Source: CAD feature listing. Evaluate the final solid. Frame: model axes, mm. A direction names the side the tool comes from. Give positions to 0.01 mm unless a question says otherwise; leave off trailing zeros. Order: outer loops, then holes, each group sorted by start corner. A loop starts at its lowest first (then second) coordinate and runs counter-clockwise, first axis right, second up. Notation, with made-up numbers: M 28,-14 L 45,-14 A12 cw 45,2 Z; hole C 9.25,20 d2. An arc over 180 degrees is marked long. Answer as a JSON object with one key per item and string values. Group by question number.
1. Section query C-C (z = -40.5). Output: boundary loops of the cut face in (x, y), plus the area to 3 significant figures.
2. Section query B-B (x = 20). Output: boundary loops of the cut face in (y, z).
3. Section query D-D (y = -7.5). Output: boundary loops of the cut face in (x, z).
4. Material intervals for L1, parallel to X at y = 2.3, z = 35.5; L2, parallel to Z at x = 40, y = 1.95; L3, parallel to X at y = 1.65, z = 90, sorted ascending. Write a range as [from, to].
5. Section query A-A (x = 0). Output: boundary loops of the cut face in (y, z).
6. Set-up query: faces 1 (the flat face through (0, -5, -95.5)), 2 (the cylindrical face through (20, 2, 65)), 3 (the flat face through (-10, -5, -93)), 4 (the flat face through (10, -5, -93)). Return all of +Z, -Z, +X, -X, +Y, -Y with unobstructed straight access to the full face (end or side cutting, diameter ignored); none if empty.
7. Pin query (flat end, axial travel): P1, Ø3.5, axis at x = 88, y = 1, coming from the -Z side; P2, Ø4, axis at x = 59, z = 69, coming from the -Y side; P3, Ø3.5, axis at x = -89, y = 2, coming from the -Z side. Return the tip coordinate at first contact, or that it passes through.
8. Pull-direction query (Z, two-part tool) for faces 5 (the flat face through (0, -5, -90.499)), 6 (the cylindrical face through (-20, 2, 15)), 7 (the flat face through (-1, 3, -24)); classes: +Z half, -Z half, draft (parallel to the pull), parting line (faces both ways), or undercut.
from build123d import *

# Parameters (mm, degrees)
SKETCH1_W               = 200
SKETCH1_H               = 200
BOSS_EXTRUDE1_DEPTH     = 3
CUT_EXTRUDE1_START      = -4
SKETCH2_W               = 30
SKETCH2_H               = 70
CUT_EXTRUDE1_DEPTH      = 14
SKETCH4_W               = 3
SKETCH4_H               = 5
CUT_EXTRUDE2_DEPTH      = 4
SKETCH5_W               = 3
SKETCH5_H               = 5
CUT_EXTRUDE3_DEPTH      = 4
CUT_EXTRUDE4_DEPTH      = 4
FILLET1_R               = 45
SKETCH9_R               = 1.5
SKETCH9_W               = 22
SKETCH9_H               = 3
CUT_EXTRUDE7_DEPTH      = 4
SKETCH11_R              = 1.5
CUT_EXTRUDE8_DEPTH      = 4
SKETCH10_R              = 1.5
CUT_EXTRUDE9_DEPTH      = 4
LPATTERN1_COUNT         = 2
LPATTERN1_PITCH         = 40
LPATTERN1_COUNT_DIR2    = 2
LPATTERN1_PITCH_DIR2    = 20
SKETCH13_R              = 1.5
CUT_EXTRUDE10_DEPTH     = 4
MIRROR1_COPY_1_SKETCH_R = 1.5
MIRROR1_COPY_1_DEPTH    = 4
MIRROR1_COPY_2_SKETCH_R = 1.5
MIRROR1_COPY_2_DEPTH    = 4
MIRROR1_COPY_3_SKETCH_R = 1.5
MIRROR1_COPY_3_DEPTH    = 4
FILLET2_R               = 0.5
SKETCH23_W              = 20
SKETCH23_H              = 5.000586006
BOSS_EXTRUDE7_DEPTH     = 10
SKETCH26_R              = 1.5
CUT_EXTRUDE11_DEPTH     = 10
SKETCH27_R              = 2.5
CUT_EXTRUDE12_DEPTH     = 10
SKETCH28_R              = 1
CUT_EXTRUDE13_DEPTH     = 10


with BuildPart() as part:
    # Sketch1 → Boss-Extrude1 (new body)
    with BuildSketch(Plane(origin=(0, 0, 0), x_dir=(1, 0, 0), z_dir=(0, 1, 0))):
        Rectangle(SKETCH1_W, SKETCH1_H)
    extrude(amount=BOSS_EXTRUDE1_DEPTH)

    # Sketch2 → Cut-Extrude1 (cut)
    with BuildSketch(Plane(origin=(0, 3, 0), x_dir=(1, 0, 0), z_dir=(0, 1, 0)).offset(CUT_EXTRUDE1_START)):
        with Locations((-85, -25)):
            Rectangle(SKETCH2_W, SKETCH2_H)
    cut_extrude1 = extrude(amount=CUT_EXTRUDE1_DEPTH, mode=Mode.SUBTRACT)

    # Sketch4 → Cut-Extrude2 (cut, through all)
    with BuildSketch(Plane(origin=(0, 3, 0), x_dir=(1, 0, 0), z_dir=(0, 1, 0))):
        with Locations((-88.5, -89.5)):
            Rectangle(SKETCH4_W, SKETCH4_H)
    cut_extrude2 = extrude(amount=-CUT_EXTRUDE2_DEPTH, mode=Mode.SUBTRACT)

    # Sketch5 → Cut-Extrude3 (cut, through all)
    with BuildSketch(Plane(origin=(0, 3, 0), x_dir=(1, 0, 0), z_dir=(0, 1, 0))):
        with Locations((-88.5, 57.5)):
            Rectangle(SKETCH5_W, SKETCH5_H)
    cut_extrude3 = extrude(amount=-CUT_EXTRUDE3_DEPTH, mode=Mode.SUBTRACT)

    # Sketch7 → Cut-Extrude4 (cut, through all)
    with BuildSketch(Plane(origin=(0, 3, 0), x_dir=(1, 0, 0), z_dir=(0, 1, 0))):
        with BuildLine():
            Line((-30, -55), (-30, -25))
            ThreePointArc((-30, -25), (-20, -15), (-10, -25))
            Line((-10, -25), (-10, -55))
            ThreePointArc((-10, -55), (-20, -65), (-30, -55))
        make_face()
    cut_extrude4 = extrude(amount=-CUT_EXTRUDE4_DEPTH, mode=Mode.SUBTRACT)

    # Fillet1
    fillet1_edges = [part.edges().sort_by_distance(p)[0] for p in [
        (-100, 1.5, -100),
        (100, 1.5, -100),
    ]]
    fillet(fillet1_edges, radius=FILLET1_R)

    # Sketch9 → Cut-Extrude7 (cut, through all)
    with BuildSketch(Plane(origin=(0, 3, 0), x_dir=(1, 0, 0), z_dir=(0, 1, 0))):
        with Locations((-60, -90)):
            Circle(SKETCH9_R)
        with BuildLine():
            Line((-30, 80), (30, 80))
            ThreePointArc((30, 80), (35, 75), (30, 70))
            Line((30, 70), (-30, 70))
            ThreePointArc((-30, 70), (-35, 75), (-30, 80))
        make_face()
        with Locations((0, 88.5)):
            Rectangle(SKETCH9_W, SKETCH9_H)
    cut_extrude7 = extrude(amount=-CUT_EXTRUDE7_DEPTH, mode=Mode.SUBTRACT)

    # Sketch11 → Cut-Extrude8 (cut, through all)
    with BuildSketch(Plane(origin=(0, 3, 0), x_dir=(1, 0, 0), z_dir=(0, 1, 0))):
        with Locations((-45, 50)):
            Circle(SKETCH11_R)
    cut_extrude8 = extrude(amount=-CUT_EXTRUDE8_DEPTH, mode=Mode.SUBTRACT)

    # Sketch10 → Cut-Extrude9 (cut, through all)
    with BuildSketch(Plane(origin=(0, 3, 0), x_dir=(1, 0, 0), z_dir=(0, 1, 0))):
        with Locations((-60, -60)):
            Circle(SKETCH10_R)
    cut_extrude9 = extrude(amount=-CUT_EXTRUDE9_DEPTH, mode=Mode.SUBTRACT)

    # LPattern1: Cut-Extrude9 2 × 2
    with Locations(*[(j * LPATTERN1_PITCH_DIR2, 0, -i * LPATTERN1_PITCH) for i in range(LPATTERN1_COUNT) for j in range(LPATTERN1_COUNT_DIR2) if (i, j) != (0, 0)]):
        add(cut_extrude9, mode=Mode.SUBTRACT)

    # Sketch13 → Cut-Extrude10 (cut, through all)
    with BuildSketch(Plane(origin=(0, 3, 0), x_dir=(1, 0, 0), z_dir=(0, 1, 0))):
        with Locations((-60, 28)):
            Circle(SKETCH13_R)
    cut_extrude10 = extrude(amount=-CUT_EXTRUDE10_DEPTH, mode=Mode.SUBTRACT)

    # Mirror1: Cut-Extrude7, Cut-Extrude10, Cut-Extrude9, Cut-Extrude8, Cut-Extrude4, Cut-Extrude3, Cut-Extrude2, Cut-Extrude1 across plane
    add(cut_extrude7.mirror(Plane(origin=(0, 0, 0), x_dir=(0, 0, 1), z_dir=(1, 0, 0))), mode=Mode.SUBTRACT)
    add(cut_extrude10.mirror(Plane(origin=(0, 0, 0), x_dir=(0, 0, 1), z_dir=(1, 0, 0))), mode=Mode.SUBTRACT)
    add(cut_extrude9.mirror(Plane(origin=(0, 0, 0), x_dir=(0, 0, 1), z_dir=(1, 0, 0))), mode=Mode.SUBTRACT)
    add(cut_extrude8.mirror(Plane(origin=(0, 0, 0), x_dir=(0, 0, 1), z_dir=(1, 0, 0))), mode=Mode.SUBTRACT)
    add(cut_extrude4.mirror(Plane(origin=(0, 0, 0), x_dir=(0, 0, 1), z_dir=(1, 0, 0))), mode=Mode.SUBTRACT)
    add(cut_extrude3.mirror(Plane(origin=(0, 0, 0), x_dir=(0, 0, 1), z_dir=(1, 0, 0))), mode=Mode.SUBTRACT)
    add(cut_extrude2.mirror(Plane(origin=(0, 0, 0), x_dir=(0, 0, 1), z_dir=(1, 0, 0))), mode=Mode.SUBTRACT)
    add(cut_extrude1.mirror(Plane(origin=(0, 0, 0), x_dir=(0, 0, 1), z_dir=(1, 0, 0))), mode=Mode.SUBTRACT)

    # Mirror1 copy 1 sketch → Mirror1 copy 1 (cut, through all)
    with BuildSketch(Plane(origin=(-20, 3, 0), x_dir=(-1, 0, 0), z_dir=(0, 1, 0))):
        with Locations((-60, 60)):
            Circle(MIRROR1_COPY_1_SKETCH_R)
    extrude(amount=-MIRROR1_COPY_1_DEPTH, mode=Mode.SUBTRACT)

    # Mirror1 copy 2 sketch → Mirror1 copy 2 (cut, through all)
    with BuildSketch(Plane(origin=(0, 3, -40), x_dir=(-1, 0, 0), z_dir=(0, 1, 0))):
        with Locations((-60, 60)):
            Circle(MIRROR1_COPY_2_SKETCH_R)
    extrude(amount=-MIRROR1_COPY_2_DEPTH, mode=Mode.SUBTRACT)

    # Mirror1 copy 3 sketch → Mirror1 copy 3 (cut, through all)
    with BuildSketch(Plane(origin=(-20, 3, -40), x_dir=(-1, 0, 0), z_dir=(0, 1, 0))):
        with Locations((-60, 60)):
            Circle(MIRROR1_COPY_3_SKETCH_R)
    extrude(amount=-MIRROR1_COPY_3_DEPTH, mode=Mode.SUBTRACT)

    # Fillet2
    fillet2_edges = [part.edges().sort_by_distance(p)[0] for p in [
        (100, 3, 80),
        (100, 3, -32.5),
        (-100, 3, 80),
        (70, 3, 25),
        (85, 3, 60),
        (85, 3, -10),
        (-70, 3, 25),
        (-85, 3, -10),
        (-85, 3, 60),
        (0, 3, 100),
        (0, 3, -100),
        (-100, 3, -32.5),
        (-86.819805153, 3, -86.819805153),
        (86.819805153, 3, -86.819805153),
    ]]
    fillet(fillet2_edges, radius=FILLET2_R)

    # Sketch23 → Boss-Extrude7 (add)
    with BuildSketch(Plane.XZ):
        with Locations((0, -92.999706997)):
            Rectangle(SKETCH23_W, SKETCH23_H)
    extrude(amount=BOSS_EXTRUDE7_DEPTH)

    # Sketch26 → Cut-Extrude11 (cut)
    with BuildSketch(Plane(origin=(0, 3, 0), x_dir=(1, 0, 0), z_dir=(0, 1, 0))):
        with Locations((24, 45.74141283)):
            Circle(SKETCH26_R)
        with Locations((-24, 45.74141283)):
            Circle(SKETCH26_R)
    extrude(amount=-CUT_EXTRUDE11_DEPTH, mode=Mode.SUBTRACT)

    # Sketch27 → Cut-Extrude12 (cut)
    with BuildSketch(Plane(origin=(0, 3, 0), x_dir=(1, 0, 0), z_dir=(0, 1, 0))):
        Circle(SKETCH27_R)
    extrude(amount=-CUT_EXTRUDE12_DEPTH, mode=Mode.SUBTRACT)

    # Sketch28 → Cut-Extrude13 (cut)
    with BuildSketch(Plane(origin=(0, 3, 0), x_dir=(1, 0, 0), z_dir=(0, 1, 0))):
        with Locations((-62.25, -35.5)):
            Circle(SKETCH28_R)
        with Locations((62.25, -35.5)):
            Circle(SKETCH28_R)
    extrude(amount=-CUT_EXTRUDE13_DEPTH, mode=Mode.SUBTRACT)


solid = part.part
Answer sheet:
{
 "1": {"outline": "M -100,0 L 100,0 L 100,2.5 A0.5 ccw 99.5,3 L -99.5,3 A0.5 ccw -100,2.5 Z", "area": "600 mm^2"},
 "2": {"outline": "M 0,-100 L 2.5,-100 A0.5 ccw 3,-99.5 L 3,-80 L 0,-80 Z; M 0,-70 L 3,-70 L 3,15 L 0,15 Z; M 0,65 L 3,65 L 3,99.5 A0.5 ccw 2.5,100 L 0,100 Z"},
 "3": {"outline": "M -10,-95.5 L 10,-95.5 L 10,-90.5 L -10,-90.5 Z"},
 "4": {"L1": "[-70, -63.25], [-61.25, -30], [-10, 10], [30, 61.25], [63.25, 70]", "L2": "[-100, 18.5], [21.5, 58.5], [61.5, 100]", "L3": "[-100, -90], [-87, -61.5], [-58.5, 58.5], [61.5, 87], [90, 100]"},
 "5": {"outline": "M -10,-95.5 L 0,-95.5 L 0,-100 L 2.5,-100 A0.5 ccw 3,-99.5 L 3,-90 L 0,-90 L 0,-90.5 L -10,-90.5 Z; M 0,-87 L 3,-87 L 3,-80 L 0,-80 Z; M 0,-70 L 3,-70 L 3,-2.5 L 0,-2.5 Z; M 0,2.5 L 3,2.5 L 3,99.5 A0.5 ccw 2.5,100 L 0,100 Z"},
 "6": {"face 1": "-Z, +X, -X, -Y", "face 2": "+Y, -Y", "face 3": "+Z, -Z, -X, -Y", "face 4": "+Z, -Z, +X, -Y"},
 "7": {"P1": "z = -87.38", "P2": "y = 0", "P3": "z = -86.38"},
 "8": {"face 5": "+Z half", "face 6": "undercut", "face 7": "draft"}
}
